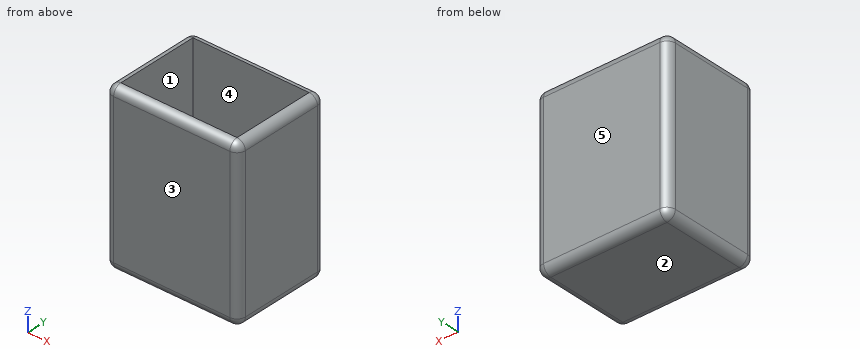
from build123d import *

# Parameters (mm, degrees)
F0_W     = 101.6
F0_H     = 76.2
F1_DEPTH = 127
F2_T     = -6.35
F3_R     = 6.34999


# Not quite as in the source:
# - a fillet or chamfer is up to 0.001 mm smaller than in the source, because OpenCascade refuses the exact size


with BuildPart() as f1:
    # F0 (on Top) → F1 (new body)
    with BuildSketch(Plane.XY):
        with Locations((-6.6963651597, -9.8136370122)):
            Rectangle(F0_W, F0_H)
    extrude(amount=F1_DEPTH)

    # F2
    f2_openings = [f1.faces().sort_by_distance(p)[0] for p in [
        (-6.696365, -9.813637, 127),
    ]]
    offset(amount=F2_T, openings=f2_openings)

    # F3 (radius 6.35 in the source; OpenCascade refuses exactly that, so slightly less here)
    f3_edges = [f1.edges().sort_by_distance(p)[0] for p in [
        (-57.496365, -47.913637, 63.5),
        (-57.496365, 28.286363, 63.5),
        (-57.496365, -9.813637, 0),
        (-57.496365, -9.813637, 127),
        (44.103635, 28.286363, 63.5),
        (-6.696365, 28.286363, 0),
        (-6.696365, 28.286363, 127),
        (44.103635, -47.913637, 63.5),
        (44.103635, -9.813637, 0),
        (44.103635, -9.813637, 127),
        (-6.696365, -47.913637, 0),
        (-6.696365, -47.913637, 127),
    ]]
    fillet(f3_edges, radius=F3_R)


solid = f1.part
The model under review builds one solid part; all positions refer to its coordinate system, in mm. Face numbers are marked on the shaded views. A direction names the side the tool comes from. Round coordinates to 2 decimals unless told otherwise and drop trailing zeros. Write each loop counter-clockwise with the first axis right and the second up, starting at its lowest first coordinate (ties: lowest second). Pieces come first, ordered by that corner, then holes. Notation, with made-up numbers: M 82,-14.75 L 128,-14.75 A20 cw 128,11.25 Z; hole C 61.25,28.25 d8. An arc over 180 degrees is marked long. Answer as CSV lines item,"result". Start each with the question number.
Q1. The part is to be moulded in two halves that separate along Y. For the marked faces 1, 2 and 3, say which applies: +Y half, -Y half, draft (parallel to the pull), parting line (faces both ways), or undercut.
Q2. Wall thickness on line 1 along Y through (x, z) = (-32, 45.5); line 2 along X through (y, z) = (-18, 13.5); line 3 along Z through (x, y) = (22, 2): over which ranges is each line inside the solid? List them lowest first.
Q3. Clearance check with a flat-ended pin moving along its axis: P1, Ø10, axis at x = 29.5, y = -9.5, coming from the +Z side. State where the tip first meets the part, or that it passes through.
Q4. Consider section A-A, the plane z = 115. Give the boundary of the cut face in (x, y).
Q5. Tool access review of the marked faces 4 and 5: name each direction out of +Z, -Z, +X, -X, +Y, -Y from which nothing blocks a thin tool from reaching the whole face with its end or side.
Result set:
1,face 1,"undercut"
1,face 2,"draft"
1,face 3,"-Y half"
2,line 1,"y = -47.91 to -41.56, 21.94 to 28.29"
2,line 2,"x = -57.5 to -51.15, 37.75 to 44.1"
2,line 3,"z = 0 to 6.35"
3,P1,"stops at z = 6.35"
4,outline,"M -57.5,-41.56 A6.35 ccw -51.15,-47.91 L 37.75,-47.91 A6.35 ccw 44.1,-41.56 L 44.1,21.94 A6.35 ccw 37.75,28.29 L -51.15,28.29 A6.35 ccw -57.5,21.94 Z; hole M -51.15,-41.56 L 37.75,-41.56 L 37.75,21.94 L -51.15,21.94 Z"
5,face 4,"+Z"
5,face 5,"+Z, -Z, +X, -X, +Y"
